Work out the finished part from the listing and answer in its coordinate system (mm). A direction names the side the tool comes from. Round coordinates to 2 decimals unless told otherwise and drop trailing zeros.
from build123d import *

# Parameters (mm, degrees)
SKETCH2_R           = 1.6
BOSS_EXTRUDE1_DEPTH = 2
SKETCH3_R           = 1.6
CUT_EXTRUDE1_DEPTH  = 10
SKETCH4_R           = 1.6
CUT_EXTRUDE2_DEPTH  = 10
CUT_EXTRUDE3_DEPTH  = 10


with BuildPart() as part:
    # Sketch2 → Boss-Extrude1 (new body)
    with BuildSketch(Plane.XY.offset(20)):
        Polygon((252.288649586, 43.377799412), (275.117398408, 93.06941092), (261.484759484, 116.375014451), (181.365813862, 123.384513926), (156.737856831, 69.776544321), (167.859011127, 50.764435642), align=None)
        with Locations((184.267611591, 120.119180009)):
            Circle(SKETCH2_R, mode=Mode.SUBTRACT)
        with Locations((270.61335305, 92.847113196)):
            Circle(SKETCH2_R, mode=Mode.SUBTRACT)
        with Locations((170.267611591, 54.568989757)):
            Circle(SKETCH2_R, mode=Mode.SUBTRACT)
    extrude(amount=BOSS_EXTRUDE1_DEPTH)

    # Sketch3 → Cut-Extrude1 (cut)
    with BuildSketch(Plane.XY.offset(22)):
        with Locations((184.767611591, 103.568989757)):
            Circle(SKETCH3_R)
        with Locations((248.767611591, 103.568989757)):
            Circle(SKETCH3_R)
        with Locations((184.767611591, 71.568989757)):
            Circle(SKETCH3_R)
        with Locations((248.767611591, 71.568989757)):
            Circle(SKETCH3_R)
    extrude(amount=-CUT_EXTRUDE1_DEPTH, mode=Mode.SUBTRACT)

    # Sketch4 → Cut-Extrude2 (cut)
    with BuildSketch(Plane.XY.offset(22)):
        with Locations((198.767683591, 105.568953757)):
            Circle(SKETCH4_R)
        with Locations((234.767611591, 105.568953757)):
            Circle(SKETCH4_R)
        with Locations((198.767683591, 69.569025757)):
            Circle(SKETCH4_R)
        with Locations((234.767611591, 69.568989757)):
            Circle(SKETCH4_R)
    extrude(amount=-CUT_EXTRUDE2_DEPTH, mode=Mode.SUBTRACT)

    # Sketch5 → Cut-Extrude3 (cut)
    with BuildSketch(Plane.XY.offset(22)):
        with BuildLine():
            Line((190.465455127, 118.196686684), (258.46886477, 112.247159259))
            ThreePointArc((258.46886477, 112.247159259), (260.532383199, 109.787953759), (258.073177698, 107.72443533))
            Line((258.073177698, 107.72443533), (190.069768055, 113.673962755))
            ThreePointArc((190.069768055, 113.673962755), (188.006249627, 116.133168256), (190.465455127, 118.196686684))
        make_face()
        with BuildLine():
            Line((181.627000542, 111.411187887), (192.965527127, 110.41919535))
            ThreePointArc((192.965527127, 110.41919535), (195.029045556, 107.959989849), (192.569840055, 105.89647142))
            Line((192.569840055, 105.89647142), (181.23131347, 106.888463958))
            ThreePointArc((181.23131347, 106.888463958), (179.167795041, 109.347669458), (181.627000542, 111.411187887))
        make_face()
        with BuildLine():
            Line((204.965527127, 109.369331387), (228.965455127, 107.269609762))
            ThreePointArc((228.965455127, 107.269609762), (231.028973556, 104.810404261), (228.569768055, 102.746885833))
            Line((228.569768055, 102.746885833), (204.569840055, 104.846607458))
            ThreePointArc((204.569840055, 104.846607458), (202.506321627, 107.305812959), (204.965527127, 109.369331387))
        make_face()
        with BuildLine():
            Line((254.965455127, 104.99490451), (263.128854265, 104.28069963))
            ThreePointArc((263.128854265, 104.28069963), (265.192372694, 101.821494129), (262.733167193, 99.7579757))
            Line((262.733167193, 99.7579757), (254.569768055, 100.472180581))
            ThreePointArc((254.569768055, 100.472180581), (252.506249627, 102.931386082), (254.965455127, 104.99490451))
        make_face()
        with BuildLine():
            Line((190.965455127, 103.035415599), (264.811196586, 96.574750372))
            ThreePointArc((264.811196586, 96.574750372), (266.874715015, 94.115544871), (264.415509514, 92.052026442))
            Line((264.415509514, 92.052026442), (190.569768055, 98.51269167))
            ThreePointArc((190.569768055, 98.51269167), (188.506249627, 100.971897171), (190.965455127, 103.035415599))
        make_face()
        with BuildLine():
            Line((174.950239512, 96.877802033), (265.772651965, 88.931870549))
            ThreePointArc((265.772651965, 88.931870549), (267.836170393, 86.472665048), (265.376964893, 84.40914662))
            Line((265.376964893, 84.40914662), (174.55455244, 92.355078103))
            ThreePointArc((174.55455244, 92.355078103), (172.491034011, 94.814283604), (174.950239512, 96.877802033))
        make_face()
        with BuildLine():
            Line((171.611858997, 89.611109106), (262.43427145, 81.665177622))
            ThreePointArc((262.43427145, 81.665177622), (264.497789879, 79.205972121), (262.038584378, 77.142453693))
            Line((262.038584378, 77.142453693), (171.216171925, 85.088385176))
            ThreePointArc((171.216171925, 85.088385176), (169.152653497, 87.547590677), (171.611858997, 89.611109106))
        make_face()
        with BuildLine():
            Line((168.277911923, 82.354066501), (242.965455127, 75.819753164))
            ThreePointArc((242.965455127, 75.819753164), (245.028973556, 73.360547663), (242.569768055, 71.297029235))
            Line((242.569768055, 71.297029235), (167.882224851, 77.831342572))
            ThreePointArc((167.882224851, 77.831342572), (165.818706422, 80.290548072), (168.277911923, 82.354066501))
        make_face()
        with BuildLine():
            Line((254.965455127, 74.769889202), (259.100324376, 74.408135017))
            ThreePointArc((259.100324376, 74.408135017), (261.163842804, 71.948929517), (258.704637304, 69.885411088))
            Line((258.704637304, 69.885411088), (254.569768055, 70.247165272))
            ThreePointArc((254.569768055, 70.247165272), (252.506249627, 72.706370773), (254.965455127, 74.769889202))
        make_face()
        with BuildLine():
            Line((164.939531408, 75.087373574), (178.965529659, 73.860257732))
            ThreePointArc((178.965529659, 73.860257732), (181.029048087, 71.401052232), (178.569842586, 69.337533803))
            Line((178.569842586, 69.337533803), (164.543844336, 70.564649645))
            ThreePointArc((164.543844336, 70.564649645), (162.480325907, 73.023855145), (164.939531408, 75.087373574))
        make_face()
        with BuildLine():
            Line((204.965527127, 71.585552702), (228.965455127, 69.485831077))
            ThreePointArc((228.965455127, 69.485831077), (231.028973556, 67.026625576), (228.569768055, 64.963107147))
            Line((228.569768055, 64.963107147), (204.569840055, 67.062828773))
            ThreePointArc((204.569840055, 67.062828773), (202.506321627, 69.522034274), (204.965527127, 71.585552702))
        make_face()
        with BuildLine():
            Line((240.965455127, 68.435967114), (255.761943861, 67.14144209))
            ThreePointArc((255.761943861, 67.14144209), (257.82546229, 64.68223659), (255.366256789, 62.618718161))
            Line((255.366256789, 62.618718161), (240.569768055, 63.913243185))
            ThreePointArc((240.569768055, 63.913243185), (238.506249627, 66.372448686), (240.965455127, 68.435967114))
        make_face()
        with BuildLine():
            Line((166.610026404, 67.382460823), (252.423563346, 59.874749163))
            ThreePointArc((252.423563346, 59.874749163), (254.487081775, 57.415543662), (252.027876274, 55.352025234))
            Line((252.027876274, 55.352025234), (166.214339332, 62.859736893))
            ThreePointArc((166.214339332, 62.859736893), (164.150820903, 65.318942394), (166.610026404, 67.382460823))
        make_face()
        with BuildLine():
            Line((176.465455127, 58.961459158), (249.085182831, 52.608056236))
            ThreePointArc((249.085182831, 52.608056236), (251.14870126, 50.148850735), (248.689495759, 48.085332307))
            Line((248.689495759, 48.085332307), (176.069768055, 54.438735229))
            ThreePointArc((176.069768055, 54.438735229), (174.006249627, 56.89794073), (176.465455127, 58.961459158))
        make_face()
    extrude(amount=-CUT_EXTRUDE3_DEPTH, mode=Mode.SUBTRACT)


solid = part.part
Q1. Find the intervals of material crossed by L1, parallel to Y at x = 170.5, z = 21.75; L2, parallel to Y at x = 270.5, z = 21.1, in increasing order.
Q2. A tool of negligible diameter and unlimited length cuts with its end or side. For faces 4 (the face through (195.033, 108.01, 21.014)), 5 (the face through (221.99, 119.83, 20.99)), from which of +Z, -Z, +X, -X, +Y, -Y can it reach the whole face along a straight path? Write none if from no direction.
Q3. The mould has two halves that part along Y. Classify faces 1 (the face through (231.033, 104.86, 21.014)), 2 (the face through (268.397, 104.559, 20.986)), 3 (the face through (209.483, 47.123, 20.986)): +Y half, -Y half, draft (parallel to the pull), parting line (faces both ways), or undercut.
Q4. Find section A-A (z = 20.3). Count the separate pieces of the cut face and the enclosed holes in it, plus the area to 3 significant figures.
Q5. Given pin 1 (5 mm diameter, centred on x = 184.77, y = 103.57, fed in from -Z); pin 2 (1.9 mm diameter, centred on x = 198.77, y = 105.57, fed in from -Z), each flat-ended and moving along its own axis, determine where each tip first touches the part or whether it passes through.
Report:
1. L1: y = 50.53 to 52.99, 56.15 to 62.48, 67.04 to 70.04, 74.6 to 77.6, 82.16 to 85.27, 89.43 to 99.73
1. L2: y = 83.02 to 91.25, 94.44 to 100.96
2. face 4: +Z, -Z
2. face 5: +Z, -Z, +X, +Y
3. face 1: undercut
3. face 2: +Y half
3. face 3: -Y half
4. separate pieces: 1
4. enclosed holes: 25
4. area: 3,900 mm2
5. pin 1: stops at z = 20
5. pin 2: passes through
